Here's the drawing with two shaded views (mm, measured from the low corner). I have some questions. A direction names the side the tool comes from. Round coordinates to 2 decimals unless told otherwise and drop trailing zeros. Loops run counter-clockwise (first coordinate to the right, second up) from the corner with the lowest first, then second, coordinate; pieces in that order, holes last. Notation, with made-up numbers: (2.5, -4) - (26.5, -4) arc R20 ccw to (26.5, 11) - close; hole circle Ø2 at (4.25, 89). An arc over 180 degrees is marked (long way). Answer as CSV lines item,"result".
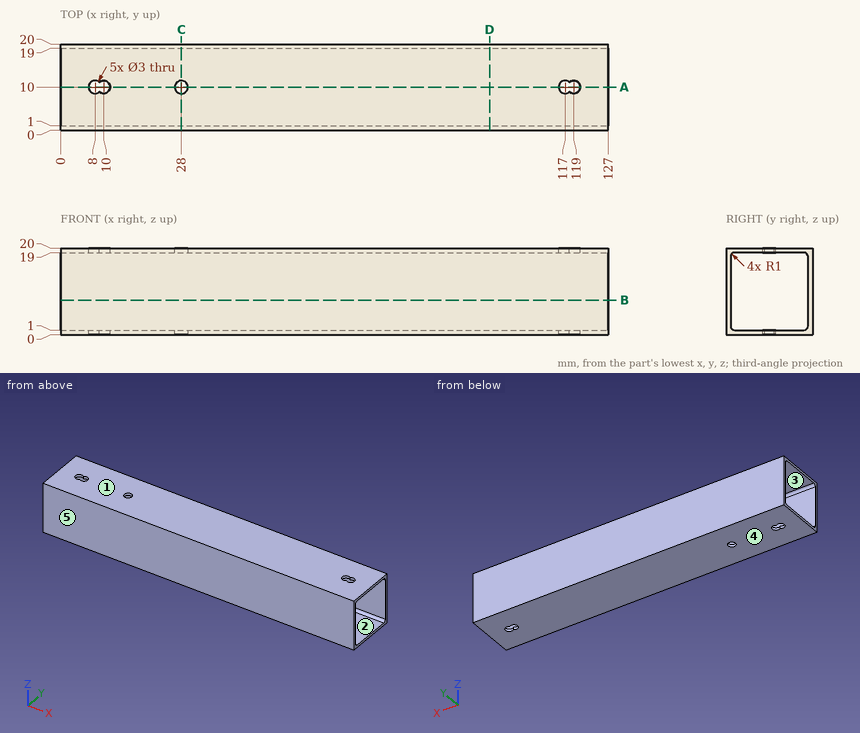
Q1. Imagine slicing it at B-B (z = 8). Write out the boundary of the cut face in (x, y), then the cut area to 3 significant figures.
Checks:
outline,"(0, 0) - (127, 0) - (127, 1) - (0, 1) - close; (0, 19) - (127, 19) - (127, 20) - (0, 20) - close"
area,"254 mm²"
Q2. If I drill on line 1 along Y through (x, z) = (119, 0.7); line 2 along Y through (x, z) = (114, 15), over which ranges is the centre line in solid material (lowest first)? Write a range as [from, to].
Checks:
line 1,"[0, 8.5], [11.5, 20]"
line 2,"[0, 1], [19, 20]"
Q3. Imagine slicing it at C-C (x = 28). Write out the boundary of the cut face in (y, z).
Checks:
outline,"(0, 0) - (8.5, 0) - (8.5, 1) - (2, 1) arc R1 cw to (1, 2) - (1, 18) arc R1 cw to (2, 19) - (8.5, 19) - (8.5, 20) - (0, 20) - close; (11.5, 0) - (20, 0) - (20, 20) - (11.5, 20) - (11.5, 19) - (18, 19) arc R1 cw to (19, 18) - (19, 2) arc R1 cw to (18, 1) - (11.5, 1) - close"
Q4. I'm going to push flat-ended pins straight in: pin 1 Ø2.5 at (x, y) = (28, 10) entering from -Z; pin 2 Ø3.5 at (x, y) = (28, 10) entering from -Z. Where does each tip first touch, or does it pass through?
Checks:
pin 1,"through"
pin 2,"z = 0"
Q5. On a 3-axis mill with a long thin cutter (end or side, diameter ignored), from which of +Z, -Z, +X, -X, +Y, -Y can I reach the whole of each face in a straight line? I mean the marked faces 1 and 2. Say none if no direction works.
Checks:
face 1,"+Z, +X, -X, +Y, -Y"
face 2,"+X, -X"
Q6. We'd pull the mould along Z, two halves only. Please class the marked faces 3, 4 and 5: pulls with the +Z half, pulls with the -Z half, needs draft (parallel to the pull), parting line crosses it, or undercut.
Checks:
face 3,"undercut"
face 4,"pulls with the -Z half"
face 5,"needs draft"
Q7. Imagine slicing it at A-A (y = 10). Count the separate pieces of the cut face and the enclosed holes in it, then the cut area to 3 significant figures.
Checks:
separate pieces,"8"
enclosed holes,"0"
area,"228 mm²"
Q8. Imagine slicing it at D-D (x = 99.5). Write out the boundary of the cut face in (y, z), then the cut area to 3 significant figures.
Checks:
outline,"(0, 0) - (20, 0) - (20, 20) - (0, 20) - close; hole (1, 2) arc R1 ccw to (2, 1) - (18, 1) arc R1 ccw to (19, 2) - (19, 18) arc R1 ccw to (18, 19) - (2, 19) arc R1 ccw to (1, 18) - close"
area,"76.9 mm²"
